For this review, take the finished solid that the model builds, in its own axes (mm). Round coordinates to 2 decimals unless told otherwise and drop trailing zeros. Loops run counter-clockwise (first coordinate to the right, second up) from the corner with the lowest first, then second, coordinate; pieces in that order, holes last.
1. Consider section A-A on z = 29. State the section outline as (x, y) points, then the cut area to 3 significant figures.
2. Clearance check with flat-ended pins moving along their axes: pin 1 Ø4 at (x, z) = (41.5, 29.5) entering from +Y (3 decimals); pin 2 Ø2 at (x, z) = (30, 13) entering from +Y. State where each tip first meets the part, or that it passes through.
3. To check wall thickness, follow line 1 along Y through (x, z) = (4, 60); line 2 along Y through (x, z) = (52, 105). State the ranges of each line that lie inside material, in increasing order.
from build123d import *

# Parameters (mm, degrees)
F0_W     = 80
F0_H     = 120
F1_DEPTH = 2700
F2_SIZE2 = 29.99999
F2_SIZE  = 119.99999
F3_SIZE2 = 119.99999
F3_SIZE  = 29.99999


# Not quite as in the source:
# - a fillet or chamfer is up to 0.001 mm smaller than in the source, because OpenCascade refuses the exact size


with BuildPart() as f1:
    # F0 (on Front) → F1 (new body)
    with BuildSketch(Plane.XZ):
        with Locations((40, 60)):
            Rectangle(F0_W, F0_H)
    extrude(amount=-F1_DEPTH)

    # F2 (size 120 and 30 in the source; OpenCascade refuses exactly that, so slightly less here)
    f2_edges = [f1.edges().sort_by_distance(p)[0] for p in [
        (40, 0, 0),
    ]]
    f2_side = f1.faces().sort_by_distance((40, 0, 60))[0]
    chamfer(f2_edges, length=F2_SIZE, length2=F2_SIZE2, reference=f2_side)

    # F3 (size 30 and 120 in the source; OpenCascade refuses exactly that, so slightly less here)
    f3_edges = [f1.edges().sort_by_distance(p)[0] for p in [
        (40, 2700, 0),
    ]]
    f3_side = f1.faces().sort_by_distance((40, 1364.999995, 0))[0]
    chamfer(f3_edges, length=F3_SIZE, length2=F3_SIZE2, reference=f3_side)


solid = f1.part
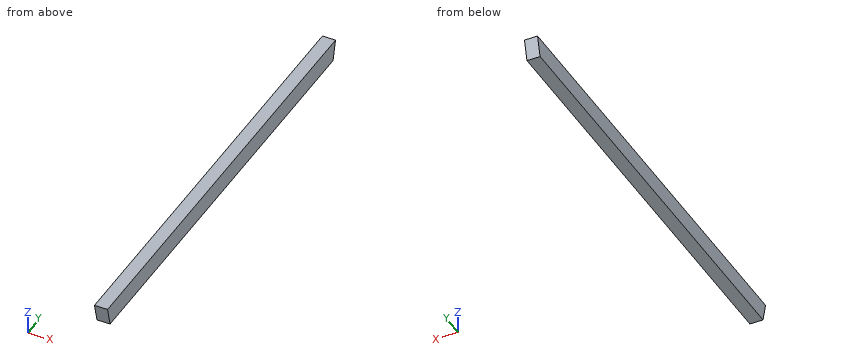
Resolved:
1. outline: (0, 22.75) - (80, 22.75) - (80, 2677.25) - (0, 2677.25) - close
1. area: 212,000 mm2
2. pin 1: stops at y = 2677.875
2. pin 2: stops at y = 2673.5
3. line 1: y = 15 to 2685
3. line 2: y = 3.75 to 2696.25
